The listing builds one solid part. Answer for the finished solid, in the listing's coordinates (mm). Face numbers are marked on the shaded views. Coordinates: 2 decimals unless noted, no trailing zeros. Order: outer loops, then holes, each group sorted by start corner. A loop starts at its lowest first (then second) coordinate and runs counter-clockwise, first axis right, second up. Notation, with made-up numbers: (88.25, 27.5) -> (138.25, 27.5) arc R34 ccw to (138.25, 60.5) -> close; hole circle Ø6 at (-15, 62.5). An arc over 180 degrees is marked (long way). Write item = value, one per line. Start each with the question number.
```python
from build123d import *

# Parameters (mm, degrees)
F0_R     = 6.985
F0_R_2   = 1.27
F1_DEPTH = 1.5875
F2_R     = 1.58749
F4_DEPTH = 0.3556
F5_COUNT = 10


# Not quite as in the source:
# - a fillet or chamfer is up to 0.001 mm smaller than in the source, because OpenCascade refuses the exact size


with BuildPart() as f1:
    # F0 (on Front) → F1 (new body, symmetric)
    with BuildSketch(Plane.XZ):
        Circle(F0_R)
        Circle(F0_R_2, mode=Mode.SUBTRACT)
    extrude(amount=F1_DEPTH, both=True)

    # F2 (radius 1.5875 in the source; OpenCascade refuses exactly that, so slightly less here)
    f2_edges = [f1.edges().sort_by_distance(p)[0] for p in [
        (-6.985, 1.5875, 0),
        (-6.985, -1.5875, 0),
    ]]
    fillet(f2_edges, radius=F2_R)

    # F3 (on Right) → F4 (join, symmetric)
    with BuildSketch(Plane.YZ):
        Polygon((-1.5832948266, 2.3071307223), (-1.4941976026, 4.4750159141), (-2.2568043449, 3.3910733182), align=None)
    f4 = extrude(amount=F4_DEPTH, both=True)

    # F5: F4 ×10 about axis
    f5_axis = Axis((0, -1.5875, 0), (0, -1, 0))
    for i in range(1, F5_COUNT):
        add(f4.rotate(f5_axis, i * 360 / F5_COUNT))


solid = f1.part
```
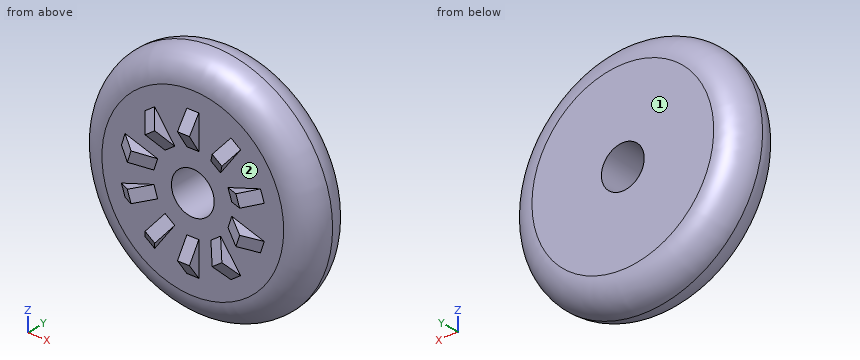
Item 1: Consider probe 1 along Z at (x, y) = (0, -0.1); probe 2 along Y at (x, z) = (0.5, 4.75); probe 3 along Z at (x, y) = (0.5, -1.15). Determine where each line is inside the solid, lowest interval first.
Item 2: Section C-C, the plane y = -0.2 is taken. Give the vertices of the cut face in (x, z), then the cut area to 3 significant figures.
Item 3: Each of these flat-tipped pins is pushed along its axis until it touches: pin 1 (0.7 mm diameter, centred on y = -2, z = -4, fed in from +X); pin 2 (2 mm diameter, centred on x = 0, z = 0, fed in from +Y); pin 3 (0.7 mm diameter, centred on y = -2, z = -3, fed in from -X); pin 4 (1.5 mm diameter, centred on x = 4, y = 0, fed in from -Z). Where does it stop, or does it pass through?
Item 4: For a pull along Z with two mould halves and no side action, classify the marked faces 1 and 2 as pulls with the +Z half, pulls with the -Z half, needs draft (parallel to the pull), parting line crosses it, or undercut.
Item 5: Section D-D, the plane y = 1.1 is taken. Give the vertices of the cut face in (x, z).
A:
q1.probe_1 = -6.98 to -1.27, 1.27 to 6.98
q1.probe_2 = -1.59 to 1.59
q1.probe_3 = -6.47 to -1.17, 1.17 to 6.47
q2.outline = circle Ø13.94 at (0, 0); hole circle Ø2.54 at (0, 0)
q2.area = 148 mm^2
q3.pin_1 = 0.36
q3.pin_2 = through
q3.pin_3 = -2.75
q3.pin_4 = -6.18
q4.face_1 = needs draft
q4.face_2 = undercut
q5.outline = circle Ø13.08 at (0, 0); hole circle Ø2.54 at (0, 0)
